Verification items for the finished model (mm, model axes). Face numbers are marked on the shaded views. Round coordinates to 2 decimals unless told otherwise and drop trailing zeros. Loops run counter-clockwise (first coordinate to the right, second up) from the corner with the lowest first, then second, coordinate; pieces in that order, holes last. Notation, with made-up numbers: M -31,58 L 5,58 A23 cw 5,78 Z; hole C 77.25,41.5 d5. An arc over 180 degrees is marked long. One line per item, written item: value.
from build123d import *

# Parameters (mm, degrees)
F0_W     = 40
F0_H     = 5
F2_SIZE  = 0.75
F3_R     = 11
F3_R_2   = 5
F4_DEPTH = 5
F7_W     = 5
F7_H     = 4
F8_DEPTH = 12.5


# Not quite as in the source:
# - a fillet or chamfer that OpenCascade refuses, or shapes differently, is made with other operations: its cross-section is extruded or revolved along the edge and cut away or added


with BuildPart() as f1:
    # F0 (on Front) → F1 (revolve)
    with BuildSketch(Plane.XZ):
        with Locations((0, 2.5)):
            Rectangle(F0_W, F0_H)
    revolve(axis=Axis((0, 0, 0), (1, 0, 0)))

    # F2
    f2_edges = [f1.edges().sort_by_distance(p)[0] for p in [
        (20, 0, -5),
    ]]
    chamfer(f2_edges, length=F2_SIZE)

    # F3 (on face) → F4 (join)
    with BuildSketch(Plane(origin=(-20, 0, 0), x_dir=(0, -1, 0), z_dir=(-1, 0, 0))):
        Circle(F3_R)
        Circle(F3_R_2, mode=Mode.SUBTRACT)
        Circle(F3_R_2)
    extrude(amount=F4_DEPTH)

    # F5: fillet of radius 11 on 1 edges, made by hand

    # F5_s1 → F5_t2 (revolve, cut)
    with BuildSketch(Plane.XY):
        with BuildLine():
            ThreePointArc((-20, -11), (-23.6695398029, -7.0244997836), (-25, -1.7804555427))
            Line((-25, -1.7804555427), (-25, -11))
            Line((-25, -11), (-20, -11))
        make_face()
    revolve(axis=Axis((-25, 0, 0), (-1, 0, 0)), mode=Mode.SUBTRACT)

    # F6: chamfer of 0.25 on 1 edges, made by hand

    # F6_s1 → F6_t2 (revolve, cut)
    with BuildSketch(Plane.XY):
        with BuildLine():
            Line((-19.9911548293, -10.7418502329), (-20.2209951465, -10.8630715284))
            Line((-20.2209951465, -10.8630715284), (-20.2238188511, -10.8671978697))
            ThreePointArc((-20.2238188511, -10.8671978697), (-20.1112438047, -10.9326533203), (-20.0027272727, -11.004190702))
            Line((-20.0027272727, -11.004190702), (-19.995, -11))
            ThreePointArc((-19.995, -11), (-19.995, -10.8709251165), (-19.9861548293, -10.7418502329))
            Line((-19.9861548293, -10.7418502329), (-19.9911548293, -10.7418502329))
        make_face()
    revolve(axis=Axis((-20, 0, 0), (-1, 0, 0)), mode=Mode.SUBTRACT)

    # F7 (on Top) → F8 (cut, symmetric)
    with BuildSketch(Plane.XY):
        with Locations((-25.2117160708, 0)):
            Rectangle(F7_W, F7_H)
    extrude(amount=F8_DEPTH, both=True, mode=Mode.SUBTRACT)


solid = f1.part
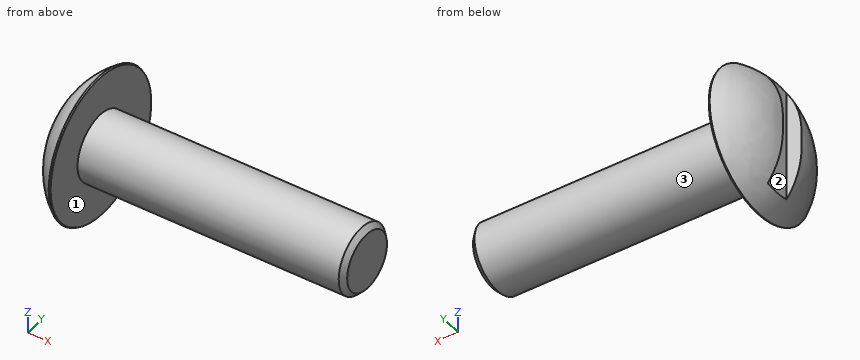
(1) Thickness scan on L1, parallel to X at y = 1, z = 2; L2, parallel to X at y = -5.75, z = -1.75; L3, parallel to Z at x = -23, y = -5.25. Record the ranges inside material, lowest first. Write a range as from..to.
Completed:
L1: x = -22.71..20
L2: x = -24.15..-20
L3: z = -6.17..6.17
(2) Depth check by flat-ended pin: pin 1 Ø1 at (x, z) = (11, 1.5) entering from -Y; pin 2 Ø4 at (x, z) = (-15, -8.5) entering from -Y; pin 3 Ø1.8 at (x, z) = (-23.5, -4) entering from -Y; pin 4 Ø1.8 at (x, z) = (-23.5, -1) entering from +Y. Enter the tip coordinate at first touch or a pass-through.
Completed:
pin 1: stops at y = -4.9
pin 2: passes through
pin 3: stops at y = -7.73
pin 4: stops at y = 8.59
(3) Mould release check, pull along Y, two halves, no side actions. Record for the marked faces 1, 2 and 3: +Y half, -Y half, draft (parallel to the pull), parting line (faces both ways), or undercut.
Completed:
face 1: draft
face 2: undercut
face 3: parting line
(4) Sectioned sample at A-A on x = -8. Enter the section's corners in (y, z), and give its area (3 significant figures).
Completed:
outline: C 0,0 d10
area: 78.5 mm^2
